Input: part model. Units: mm. Frame: model coordinates. Give positions to 0.01 mm unless a question says otherwise; leave off trailing zeros. Loops run counter-clockwise (first coordinate to the right, second up) from the corner with the lowest first, then second, coordinate; pieces in that order, holes last. Notation, with made-up numbers: M -17.75,37 L 5.25,37 A22 cw 5.25,45 Z; hole C 16.25,39 d2. An arc over 180 degrees is marked long. Use CSV: the item, a comma, the result in double quotes. Start each with the question number.
Q1. Material intervals for line 1 along Z through (x, y) = (98.5, -3); line 2 along Y through (x, z) = (105.5, -6); line 3 along Y through (x, z) = (-136, 0), sorted ascending.
Q2. Pin query (flat end, axial travel): pin 1 (5 mm diameter, centred on x = -116, y = -6, fed in from -Z); pin 2 (0.7 mm diameter, centred on x = 67, z = -7.5, fed in from +Y); pin 3 (3 mm diameter, centred on x = 128, y = -3.5, fed in from +Z); pin 4 (4.5 mm diameter, centred on x = 41.5, z = 0, fed in from -Y). Return the tip coordinate at first contact, or that it passes through.
Q3. Section A-A, the plane x = -82. Output: boundary loops of the cut face in (y, z).
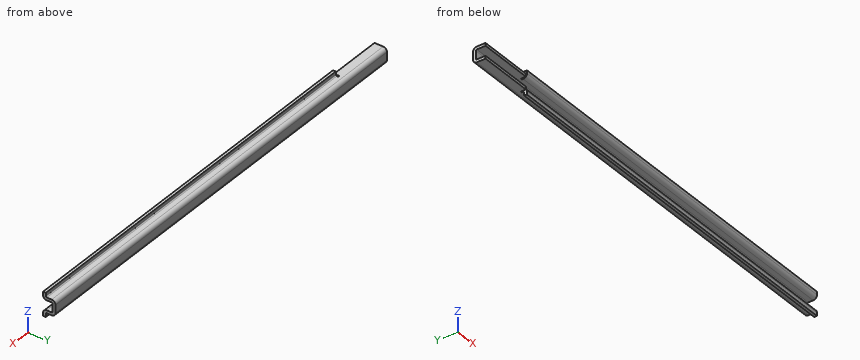
from build123d import *

# Parameters (mm, degrees)
SKETCH2_W                       = 322.4
SKETCH2_H                       = 11
BASE_FLANGE1_DEPTH              = 2
EDGE_FLANGE1_STRIP_W            = 9.4732
EDGE_FLANGE1_STRIP_H            = 2
EDGE_FLANGE1_STRIP_CUT_DEPTH    = 322.4
EDGE_FLANGE1_STRIP_2_W          = 9.4732
EDGE_FLANGE1_STRIP_2_H          = 2
EDGE_FLANGE1_STRIP_CUT_2_DEPTH  = 322.4
EDGE_FLANGE1_DEPTH              = 322.4
EDGE_FLANGE1_BEND_DEPTH         = 322.4
EDGE_FLANGE3_STRIP_W            = 9.4732
EDGE_FLANGE3_STRIP_H            = 2
EDGE_FLANGE3_STRIP_CUT_DEPTH    = 282.1
EDGE_FLANGE3_RELIEF_W           = 10.4732
EDGE_FLANGE3_RELIEF_H           = 1
EDGE_FLANGE3_RELIEF_CUT_DEPTH   = 2
EDGE_FLANGE3_STRIP_2_W          = 9.4732
EDGE_FLANGE3_STRIP_2_H          = 2
EDGE_FLANGE3_STRIP_CUT_2_DEPTH  = 282.1
EDGE_FLANGE3_RELIEF_2_W         = 10.4732
EDGE_FLANGE3_RELIEF_2_H         = 1
EDGE_FLANGE3_RELIEF_CUT_2_DEPTH = 2
EDGE_FLANGE3_DEPTH              = 282.1
EDGE_FLANGE3_BEND_DEPTH         = 282.1


# Sheet-metal steps are written as plain solids
with BuildPart() as part:
    # Sketch2 → Base-Flange1 (new body)
    with BuildSketch(Plane(origin=(0, 0, 0), x_dir=(1, 0, 0), z_dir=(0, 1, 0))):
        Rectangle(SKETCH2_W, SKETCH2_H)
    extrude(amount=-BASE_FLANGE1_DEPTH)

    # Edge-Flange1 strip (across the edge) → Edge-Flange1 strip cut (cut)
    with BuildSketch(Plane(origin=(161.2, -2, 5.5), x_dir=(0, 0, -1), z_dir=(-1, 0, 0))):
        with Locations((-2, -1)):
            Rectangle(EDGE_FLANGE1_STRIP_W, EDGE_FLANGE1_STRIP_H)
    extrude(amount=EDGE_FLANGE1_STRIP_CUT_DEPTH, mode=Mode.SUBTRACT)

    # Edge-Flange1 strip 2 (across the edge) → Edge-Flange1 strip cut 2 (cut)
    with BuildSketch(Plane(origin=(-161.2, -2, -5.5), x_dir=(0, 0, 1), z_dir=(1, 0, 0))):
        with Locations((-2, -1)):
            Rectangle(EDGE_FLANGE1_STRIP_2_W, EDGE_FLANGE1_STRIP_2_H)
    extrude(amount=EDGE_FLANGE1_STRIP_CUT_2_DEPTH, mode=Mode.SUBTRACT)

    # Edge-Flange1 section (across the edge) → Edge-Flange1 (add)
    with BuildSketch(Plane(origin=(161.2, -2, 5.5), x_dir=(0, 0, -1), z_dir=(-1, 0, 0))):
        with BuildLine():
            Line((0, 0.7366), (0, 7))
            Line((0, 7), (2, 7))
            Line((2, 7), (2, 0.7366))
            ThreePointArc((2, 0.7366), (2.215745145, 0.215745145), (2.7366, 0))
            Line((2.7366, 0), (2.7366, -2))
            ThreePointArc((2.7366, -2), (0.801531583, -1.198468417), (0, 0.7366))
        make_face()
    extrude(amount=EDGE_FLANGE1_DEPTH)

    # Edge-Flange1 section 2 (across the edge) → Edge-Flange1 bend (add)
    with BuildSketch(Plane(origin=(-161.2, -2, -5.5), x_dir=(0, 0, 1), z_dir=(1, 0, 0))):
        with BuildLine():
            Line((0, 0.7366), (0, 7))
            Line((0, 7), (2, 7))
            Line((2, 7), (2, 0.7366))
            ThreePointArc((2, 0.7366), (2.215745145, 0.215745145), (2.7366, 0))
            Line((2.7366, 0), (2.7366, -2))
            ThreePointArc((2.7366, -2), (0.801531583, -1.198468417), (0, 0.7366))
        make_face()
    extrude(amount=EDGE_FLANGE1_BEND_DEPTH)

    # Edge-Flange3 strip (across the edge) → Edge-Flange3 strip cut (cut)
    with BuildSketch(Plane(origin=(-120.9, -9, 5.5), x_dir=(0, 1, 0), z_dir=(1, 0, 0))):
        with Locations((-2, -1)):
            Rectangle(EDGE_FLANGE3_STRIP_W, EDGE_FLANGE3_STRIP_H)
    extrude(amount=EDGE_FLANGE3_STRIP_CUT_DEPTH, mode=Mode.SUBTRACT)

    # Edge-Flange3 relief (on the sheet) → Edge-Flange3 relief cut (cut)
    with BuildSketch(Plane(origin=(-120.9, -6.2634, 5.5), x_dir=(0, 1, 0), z_dir=(0, 0, 1))):
        with Locations((-4.2366, 0.5)):
            Rectangle(EDGE_FLANGE3_RELIEF_W, EDGE_FLANGE3_RELIEF_H)
    extrude(amount=-EDGE_FLANGE3_RELIEF_CUT_DEPTH, mode=Mode.SUBTRACT)

    # Edge-Flange3 strip 2 (across the edge) → Edge-Flange3 strip cut 2 (cut)
    with BuildSketch(Plane(origin=(161.2, -9, -5.5), x_dir=(0, 1, 0), z_dir=(-1, 0, 0))):
        with Locations((-2, -1)):
            Rectangle(EDGE_FLANGE3_STRIP_2_W, EDGE_FLANGE3_STRIP_2_H)
    extrude(amount=EDGE_FLANGE3_STRIP_CUT_2_DEPTH, mode=Mode.SUBTRACT)

    # Edge-Flange3 relief 2 (on the sheet) → Edge-Flange3 relief cut 2 (cut)
    with BuildSketch(Plane(origin=(161.2, -6.2634, -5.5), x_dir=(0, 1, 0), z_dir=(0, 0, -1))):
        with Locations((-4.2366, -282.6)):
            Rectangle(EDGE_FLANGE3_RELIEF_2_W, EDGE_FLANGE3_RELIEF_2_H)
    extrude(amount=-EDGE_FLANGE3_RELIEF_CUT_2_DEPTH, mode=Mode.SUBTRACT)

    # Edge-Flange3 section (across the edge) → Edge-Flange3 (add)
    with BuildSketch(Plane(origin=(-120.9, -9, 5.5), x_dir=(0, 1, 0), z_dir=(1, 0, 0))):
        with BuildLine():
            Line((0, 0.7366), (0, 3))
            Line((0, 3), (2, 3))
            Line((2, 3), (2, 0.7366))
            ThreePointArc((2, 0.7366), (2.215745145, 0.215745145), (2.7366, 0))
            Line((2.7366, 0), (2.7366, -2))
            ThreePointArc((2.7366, -2), (0.801531583, -1.198468417), (0, 0.7366))
        make_face()
    extrude(amount=EDGE_FLANGE3_DEPTH)

    # Edge-Flange3 section 2 (across the edge) → Edge-Flange3 bend (add)
    with BuildSketch(Plane(origin=(161.2, -9, -5.5), x_dir=(0, 1, 0), z_dir=(-1, 0, 0))):
        with BuildLine():
            Line((0, 0.7366), (0, 3))
            Line((0, 3), (2, 3))
            Line((2, 3), (2, 0.7366))
            ThreePointArc((2, 0.7366), (2.215745145, 0.215745145), (2.7366, 0))
            Line((2.7366, 0), (2.7366, -2))
            ThreePointArc((2.7366, -2), (0.801531583, -1.198468417), (0, 0.7366))
        make_face()
    extrude(amount=EDGE_FLANGE3_BEND_DEPTH)


solid = part.part
A:
1,line 1,"-5.5 to -3.5, 3.5 to 5.5"
1,line 2,"-8.99 to -6.96"
1,line 3,"-2 to 0"
2,pin 1,"z = -8.5"
2,pin 2,"y = -7"
2,pin 3,"z = 5.5"
2,pin 4,"y = -2"
3,outline,"M -9,-8.5 L -7,-8.5 L -7,-6.24 A0.74 cw -6.26,-5.5 L -2.74,-5.5 A2.74 ccw 0,-2.76 L 0,2.76 A2.74 ccw -2.74,5.5 L -6.26,5.5 A0.74 cw -7,6.24 L -7,8.5 L -9,8.5 L -9,6.24 A2.74 ccw -6.26,3.5 L -2.74,3.5 A0.74 cw -2,2.76 L -2,-2.76 A0.74 cw -2.74,-3.5 L -6.26,-3.5 A2.74 ccw -9,-6.24 Z"
